```python
from build123d import *

# Parameters (mm, degrees)
SKETCH_W          = 28.4
SKETCH_H          = 28.4
PAD_DEPTH         = 175
SKETCH001_R       = 6.4
POCKET_DEPTH      = 175.001
POCKET_DEPTH_BACK = -0.001
SKETCH002_R       = 2.74807
POCKET001_DEPTH   = 0.1
SKETCH003_W       = 35
SKETCH003_H       = 35
PAD001_DEPTH      = 15
FILLET_R          = 3
CHAMFER_SIZE      = 3
FILLET001_R       = 3
FILLET002_R       = 5
FILLET003_R       = 7
FILLET004_R       = 1
POCKET002_DEPTH   = 31.701
POCKET003_DEPTH   = 31.701
SKETCH006_R       = 6.4
POCKET004_DEPTH   = 190.001


with BuildPart() as part:
    # Sketch → Pad (new body)
    with BuildSketch(Plane.XY):
        Rectangle(SKETCH_W, SKETCH_H)
    extrude(amount=PAD_DEPTH)

    # Sketch001 → Pocket (cut, two sides)
    with BuildSketch(Plane(origin=(0, 0, 0), x_dir=(1, 0, 0), z_dir=(0, 0, -1))) as pocket_sk:
        Circle(SKETCH001_R)
    extrude(amount=-POCKET_DEPTH, mode=Mode.SUBTRACT)
    extrude(pocket_sk.sketch, amount=-POCKET_DEPTH_BACK, mode=Mode.SUBTRACT)

    # Sketch002 → Pocket001 (cut)
    with BuildSketch(Plane.YZ.offset(14.2)):
        with Locations((0, 131.580032)):
            Circle(SKETCH002_R)
    extrude(amount=-POCKET001_DEPTH, mode=Mode.SUBTRACT)

    # Sketch003 → Pad001 (new body)
    with BuildSketch(Plane(origin=(0, 0, 0), x_dir=(1, 0, 0), z_dir=(0, 0, -1))):
        Rectangle(SKETCH003_W, SKETCH003_H)
    extrude(amount=PAD001_DEPTH)

    # Fillet
    fillet_edges = [part.edges().sort_by_distance(p)[0] for p in [
        (17.5, -17.5, -7.5),
        (-17.5, -17.5, -7.5),
        (17.5, 17.5, -7.5),
        (-17.5, 17.5, -7.5),
    ]]
    fillet(fillet_edges, radius=FILLET_R)

    # Chamfer
    chamfer_edges = [part.edges().sort_by_distance(p)[0] for p in [
        (0, -17.5, -15),
        (-16.62132, -16.62132, -15),
        (16.62132, -16.62132, -15),
        (-17.5, 0, -15),
        (17.5, 0, -15),
        (-16.62132, 16.62132, -15),
        (16.62132, 16.62132, -15),
        (0, 17.5, -15),
    ]]
    chamfer(chamfer_edges, length=CHAMFER_SIZE)

    # Fillet001
    fillet001_edges = [part.edges().sort_by_distance(p)[0] for p in [
        (14.2, -14.2, 87.5),
        (14.2, 14.2, 87.5),
        (-14.2, 14.2, 87.5),
        (-14.2, -14.2, 87.5),
    ]]
    fillet(fillet001_edges, radius=FILLET001_R)

    # Fillet002
    fillet002_edges = [part.edges().sort_by_distance(p)[0] for p in [
        (14.2, 0, 175),
    ]]
    fillet(fillet002_edges, radius=FILLET002_R)

    # Fillet003
    fillet003_edges = [part.edges().sort_by_distance(p)[0] for p in [
        (17.5, 0, -12),
    ]]
    fillet(fillet003_edges, radius=FILLET003_R)

    # Fillet004
    fillet004_edges = [part.edges().sort_by_distance(p)[0] for p in [
        (0, 17.5, 0),
    ]]
    fillet(fillet004_edges, radius=FILLET004_R)

    # Sketch004 → Pocket002 (cut, through all)
    with BuildSketch(Plane(origin=(0, 14.2, 0), x_dir=(-1, 0, 0), z_dir=(0, 1, 0))):
        Polygon((0, 34.242641), (-4.242641, 30), (0, 25.757359), (4.242641, 30), align=None)
    extrude(amount=-POCKET002_DEPTH, mode=Mode.SUBTRACT)

    # Sketch005 → Pocket003 (cut, through all)
    with BuildSketch(Plane(origin=(-14.2, 0, 0), x_dir=(0, -1, 0), z_dir=(-1, 0, 0))):
        Polygon((0, 161.242641), (-4.242641, 157), (0, 152.757359), (4.242641, 157), align=None)
    extrude(amount=-POCKET003_DEPTH, mode=Mode.SUBTRACT)

    # Sketch006 → Pocket004 (cut, through all)
    with BuildSketch(Plane(origin=(0, 0, -15), x_dir=(1, 0, 0), z_dir=(0, 0, -1))):
        Circle(SKETCH006_R)
    extrude(amount=-POCKET004_DEPTH, mode=Mode.SUBTRACT)


solid = part.part
```
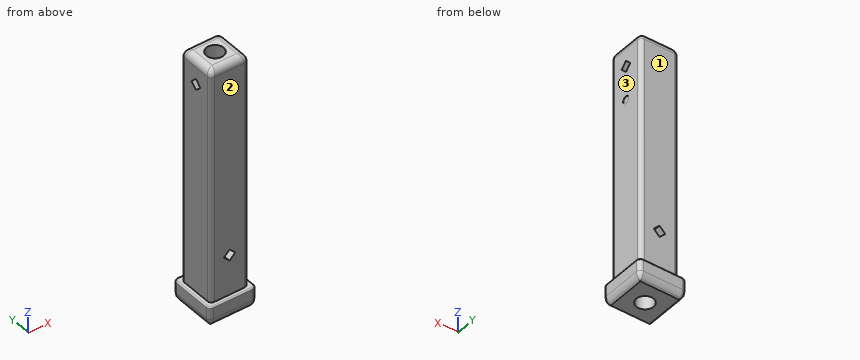
Design review of the part built by this model. Coordinates are the model's own, in mm. Face numbers are marked on the shaded views. A direction names the side the tool comes from. Give positions to 0.01 mm unless a question says otherwise; leave off trailing zeros. Order: outer loops, then holes, each group sorted by start corner. A loop starts at its lowest first (then second) coordinate and runs counter-clockwise, first axis right, second up. Notation, with made-up numbers: M -8.75,40.5 L 39.25,40.5 A13 ccw 39.25,60.5 Z; hole C 45.5,62.5 d1. An arc over 180 degrees is marked long. One line per question, with ' | ' between items. Start each with the question number.
Q1. For L1, parallel to X at y = 0, z = 82; L2, parallel to X at y = -8.5, z = 25, list the stretches that pass through material, from the lowest coordinate up. Write a range as [from, to].
Q2. We need section A-A (z = 68). Write out the cut boundary in (x, y), plus the area to 3 significant figures.
Q3. Machinability: for the marked faces 1, 2 and 3, which of the approach directions +Z, -Z, +X, -X, +Y, -Y give a long, thin tool a straight path to every point of the face, cutting with its end or side? Answer none if there is none.
Q4. For pin 1 Ø1.5 at (y, z) = (-4.5, 94) entering from +X; pin 2 Ø6.5 at (x, z) = (-3, 109.5) entering from -Y; pin 3 Ø6.5 at (y, z) = (5, 95) entering from -X, all flat-tipped, find the tip position at first contact; note any pin that passes through.
Returned:
1) L1: [-14.2, -6.4], [6.4, 14.2] | L2: [-14.2, 14.2]
2) outline: M -14.2,-11.2 A3 ccw -11.2,-14.2 L 11.2,-14.2 A3 ccw 14.2,-11.2 L 14.2,11.2 A3 ccw 11.2,14.2 L -11.2,14.2 A3 ccw -14.2,11.2 Z; hole C 0,0 d12.8 | area: 670 mm2
3) face 1: +Z, +X, -X, +Y | face 2: +Z, +X, -X, -Y | face 3: +Z, +X, +Y, -Y
4) pin 1: x = 14.2 | pin 2: y = -14.2 | pin 3: x = -14.2
